Read the model definition and answer for the solid it produces. Units are mm, in the model's axes. Face numbers are marked on the shaded views. A direction names the side the tool comes from. Coordinates: 2 decimals unless noted, no trailing zeros. Loops run counter-clockwise (first coordinate to the right, second up) from the corner with the lowest first, then second, coordinate; pieces in that order, holes last. Notation, with made-up numbers: (8, -29.5) - (44, -29.5) arc R4 ccw to (44, -25.5) - close; hole circle Ø7 at (72.5, -13). An arc over 180 degrees is marked (long way). Use one line per item in the form item = value. Start each with the question number.
1) A cutting plane is placed at D-D (x = 29). Give the vertices of the cut face in (y, z).
2) Which of the six approach directions +Z, -Z, +X, -X, +Y, -Y give full straight-line access (tool end or side, diameter ignored) to the marked faces 1, 2, 3 and 4?
3) Each of these flat-tipped pins is pushed along its axis until it touches: P1, Ø4, axis at x = 34.5, y = 8.5, coming from the +Z side; P2, Ø0.8, axis at y = 2.5, z = -6.5, coming from the -X side; P3, Ø0.8, axis at y = 3, z = 7, coming from the -X side. Where does it stop, or does it pass through?
4) A cutting plane is placed at A-A (x = -5.25). Give the vertices of the cut face in (y, z).
5) A cutting plane is placed at C-C (z = 2.5). Give the vertices of the cut face in (x, y), and give its area (3 significant figures).
6) Consider line 1 (X direction, y = 1, z = 0); line 2 (Z direction, x = 83, y = 16.25); line 3 (X direction, y = 1, z = -8.5) (3 decimals). Determine where each line is inside the solid, lowest interval first.
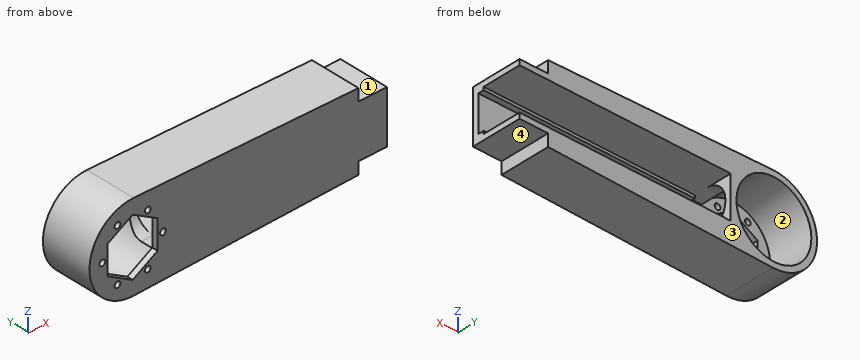
from build123d import *

# Parameters (mm, degrees)
BOSS_EXTRUDE1_DEPTH     = 17.5
SKETCH2_W               = 252
SKETCH2_H               = 14.5
CUT_EXTRUDE1_DEPTH      = 15.5
SKETCH3_R               = 13
CUT_EXTRUDE2_DEPTH      = 15.5
CUT_EXTRUDE3_REACH      = 264.265
CUT_EXTRUDE3_END_RADIUS = 13
SKETCH5_W               = 252
SKETCH5_H               = 1
BOSS_EXTRUDE2_DEPTH     = 2
SKETCH6_R               = 1
CUT_EXTRUDE4_DEPTH      = 2
CUT_EXTRUDE9_DEPTH      = 278.209870862


with BuildPart() as part:
    # Sketch1 → Boss-Extrude1 (new body)
    with BuildSketch(Plane(origin=(0, 0, 0), x_dir=(1, 0, 0), z_dir=(0, 1, 0))):
        with BuildLine():
            Line((0.323033708, 14.996521237), (267.19920412, 9.247854763))
            ThreePointArc((267.19920412, 9.247854763), (276.25, 0), (267.19920412, -9.247854763))
            Line((267.19920412, -9.247854763), (0.323033708, -14.996521237))
            ThreePointArc((0.323033708, -14.996521237), (-15, 0), (0.323033708, 14.996521237))
        make_face()
    extrude(amount=BOSS_EXTRUDE1_DEPTH)

    # Sketch2 → Cut-Extrude1 (cut)
    with BuildSketch(Plane(origin=(0, 17.5, 0), x_dir=(1, 0, 0), z_dir=(0, 1, 0))):
        with Locations((141, 0)):
            Rectangle(SKETCH2_W, SKETCH2_H)
    extrude(amount=-CUT_EXTRUDE1_DEPTH, mode=Mode.SUBTRACT)

    # Sketch3 → Cut-Extrude2 (cut)
    with BuildSketch(Plane(origin=(0, 17.5, 0), x_dir=(1, 0, 0), z_dir=(0, 1, 0))):
        with Locations(Location((0, 0, 0), (0, 0, 270))):
            Circle(SKETCH3_R)
    extrude(amount=-CUT_EXTRUDE2_DEPTH, mode=Mode.SUBTRACT)

    # Cut-Extrude3: up to this cylinder (the profile starts outside it)
    cut_extrude3_end = Plane(origin=(0, 8.125709, 0), z_dir=(0, 1, 0)) * Cylinder(CUT_EXTRUDE3_END_RADIUS, 555.53, mode=Mode.PRIVATE)
    # Sketch4 → Cut-Extrude3 (cut, up to the surface)
    with BuildSketch(Plane(origin=(15, 0, 0), x_dir=(0, 0, -1), z_dir=(1, 0, 0)), mode=Mode.PRIVATE) as cut_extrude3_sk1:
        with BuildLine():
            Line((-7.25, 2), (7.25, 2))
            Line((7.25, 2), (7.25, 8.5))
            ThreePointArc((7.25, 8.5), (5.199747468, 13.449747468), (0.25, 15.5))
            Line((0.25, 15.5), (-0.25, 15.5))
            ThreePointArc((-0.25, 15.5), (-5.199747468, 13.449747468), (-7.25, 8.5))
            Line((-7.25, 8.5), (-7.25, 2))
        make_face()
    cut_extrude3_tool1 = extrude(cut_extrude3_sk1.sketch, amount=-CUT_EXTRUDE3_REACH, mode=Mode.PRIVATE) - cut_extrude3_end
    add(cut_extrude3_tool1.solids().sort_by_distance((15, 8.125709, 0))[0], mode=Mode.SUBTRACT)

    # Sketch5 → Boss-Extrude2 (add)
    with BuildSketch(Plane(origin=(0, 2, 0), x_dir=(1, 0, 0), z_dir=(0, 1, 0))):
        with Locations((141, 6.75)):
            Rectangle(SKETCH5_W, SKETCH5_H)
        with Locations((141, -6.75)):
            Rectangle(SKETCH5_W, SKETCH5_H)
    extrude(amount=BOSS_EXTRUDE2_DEPTH)

    # Sketch6 → Cut-Extrude4 (cut)
    with BuildSketch(Plane(origin=(0, 2, 0), x_dir=(1, 0, 0), z_dir=(0, 1, 0))):
        with Locations(Location((-5.25, 9.09326674, 0), (0, 0, 270))):
            Circle(SKETCH6_R)
        with Locations(Location((-10.5, 0, 0), (0, 0, 270))):
            Circle(SKETCH6_R)
        with Locations(Location((5.25, 9.09326674, 0), (0, 0, 270))):
            Circle(SKETCH6_R)
        with Locations(Location((10.5, 0, 0), (0, 0, 270))):
            Circle(SKETCH6_R)
        with Locations(Location((5.25, -9.09326674, 0), (0, 0, 270))):
            Circle(SKETCH6_R)
        with Locations(Location((-5.25, -9.09326674, 0), (0, 0, 270))):
            Circle(SKETCH6_R)
        Polygon((0, -10), (8.660254038, -5), (8.660254038, 5), (0, 10), (-8.660254038, 5), (-8.660254038, -5), align=None)
    extrude(amount=-CUT_EXTRUDE4_DEPTH, mode=Mode.SUBTRACT)

    # Sketch14 → Cut-Extrude9 (cut, through all)
    with BuildSketch(Plane(origin=(0, 0, 0), x_dir=(1, 0, 0), z_dir=(0, 1, 0))):
        Polygon((88.5, 9.35), (78.6, 9.35), (78.6, 35), (78.4, 35), (78.4, 9.15), (88.3, 9.15), (88.3, -9.15), (78.4, -9.15), (78.4, -35), (78.6, -35), (78.6, -9.35), (88.5, -9.35), align=None)
        Polygon((172.7, 9.15), (182.6, 9.15), (182.6, 35), (182.4, 35), (182.4, 9.35), (172.5, 9.35), (172.5, 9.25), (172.5, -9.35), (182.4, -9.35), (182.4, -35), (182.6, -35), (182.6, -9.15), (172.7, -9.15), align=None)
    extrude(amount=CUT_EXTRUDE9_DEPTH, mode=Mode.SUBTRACT)


with BuildPart() as cut_extrude9_kept_piece:
    # of the separate pieces the step leaves, the one the design keeps (cut_extrude9_pieces_kept)
    add(part.part.solids().sort_by_distance((78.4, 0, 13.314698399))[0])


solid = cut_extrude9_kept_piece.part
Found:
q1.outline = (0, -14.38) - (17.5, -14.38) - (17.5, -7.25) - (4, -7.25) - (4, -6.25) - (2, -6.25) - (2, 6.25) - (4, 6.25) - (4, 7.25) - (17.5, 7.25) - (17.5, 14.38) - (0, 14.38) - close
q2.face_1 = +Z, +X, +Y, -Y
q2.face_2 = +Y
q2.face_3 = +Z, -Z, +X, -X, +Y
q2.face_4 = -Z, +X, +Y, -Y
q3.P1 = 14.3
q3.P2 = -13.7
q3.P3 = -13.47
q4.outline = (0, -14.05) - (17.5, -14.05) - (17.5, -11.89) - (2, -11.89) - (2, -10.09) - (0, -10.09) - close; (0, -8.09) - (2, -8.09) - (2, -6.97) - (0, -6.97) - close; (0, 6.97) - (2, 6.97) - (2, 8.09) - (0, 8.09) - close; (0, 10.09) - (2, 10.09) - (2, 11.89) - (17.5, 11.89) - (17.5, 14.05) - (0, 14.05) - close
q5.outline = (-14.79, 0) - (-8.66, 0) - (-8.66, 2) - (-12.76, 2) - (-12.76, 17.5) - (-14.79, 17.5) - close; (8.66, 0) - (88.3, 0) - (88.3, 2) - (8.66, 2) - close; (12.76, 15.13) - (15, 15.13) - (15, 17.5) - (12.76, 17.5) - close
q5.area = 208 mm^2
q6.line_1 = -15 to -11.5, -9.5 to -8.66, 8.66 to 9.5, 11.5 to 88.3
q6.line_2 = -9.15 to -7.25, 7.25 to 9.15
q6.line_3 = -12.359 to -6.055, -4.445 to -2.598, 2.598 to 4.445, 6.055 to 88.3
